Here's how the part is built. I have some questions about the finished solid (model axes, mm). Face numbers are marked on the shaded views. A direction names the side the tool comes from. Coordinates: 2 decimals unless noted, no trailing zeros. Order: outer loops, then holes, each group sorted by start corner. A loop starts at its lowest first (then second) coordinate and runs counter-clockwise, first axis right, second up. Notation, with made-up numbers: (18, 57.5) - (31, 57.5) arc R29 ccw to (31, 85.5) - close; hole circle Ø10 at (60.25, 15). An arc over 180 degrees is marked (long way). Answer as CSV lines item,"result". Start each with the question number.
Item 1: I need wall thicknesses on line 1 (X direction, y = 1.2, z = 4.5) (3 decimals); line 2 (X direction, y = 1.45, z = 31.5) (3 decimals); line 3 (X direction, y = 10.5, z = 6.5). Which ranges of each line are inside material? Lowest first, please.
Item 2: On a 3-axis mill with a long thin cutter (end or side, diameter ignored), from which of +Z, -Z, +X, -X, +Y, -Y can I reach the whole of each face in a straight line? I mean the marked faces 1, 2, 3 and 4. Say none if no direction works.
Item 3: Imagine slicing it at C-C on x = 4.5. List the corners of the cut face in (y, z) for me (3 decimals).
Item 4: Imagine slicing it at A-A on z = 29. List the corners of the cut face in (x, y) for me, and give its area (3 significant figures).
Item 5: I'm going to push flat-ended pins straight in: pin 1 (3.5 mm diameter, centred on y = 7.5, z = 18, fed in from +X); pin 2 (1.5 mm diameter, centred on y = 7, z = 6.5, fed in from -X); pin 3 (3.5 mm diameter, centred on x = 36, z = 11, fed in from +Y); pin 4 (1.5 mm diameter, centred on x = 29.5, y = 2, fed in from -Z). Where does each tip first touch, or does it pass through?
Item 6: Imagine slicing it at D-D on z = 16. List the corners of the cut face in (x, y) for me.
Item 7: We'd pull the mould along X, two halves only. Please class the marked faces 5 and 6: pulls with the +X half, pulls with the -X half, needs draft (parallel to the pull), parting line crosses it, or undercut.
Item 8: Imagine slicing it at B-B on y = 7.5. List the corners of the cut face in (x, z) for me.
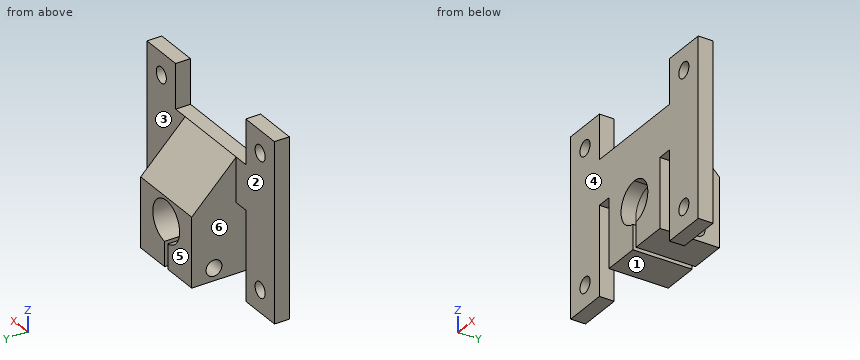
from build123d import *

# Parameters (mm, degrees)
SKETCH2_R           = 1.575
BOSS_EXTRUDE4_DEPTH = 3
BOSS_EXTRUDE5_DEPTH = 9
RIB2_REACH          = 44.895
SKETCH8_WALL_W      = 100.51836442
SKETCH8_WALL_H      = 16
SKETCH9_R           = 1.6
CUT_EXTRUDE1_DEPTH  = 48.15930449


with BuildPart() as part:
    # Sketch2 → Boss-Extrude4 (new body)
    # profile 1 of 4: a face of its own
    with BuildSketch(Plane(origin=(0, 0, 0), x_dir=(1, 0, 0), z_dir=(0, 1, 0))):
        Polygon((28, -18), (20, -18), (20, -27), (31, -27), (31, -36), (40, -36), (40, 0), (31, 0), (31, -18), align=None)
        with Locations(Location((35.5, -31.5, 0), (0, 0, 270))):
            Circle(SKETCH2_R, mode=Mode.SUBTRACT)
        with Locations(Location((35.5, -4.5, 0), (0, 0, 270))):
            Circle(SKETCH2_R, mode=Mode.SUBTRACT)
    # profile 2 of 4: a face of its own
    with BuildSketch(Plane(origin=(0, 0, 0), x_dir=(1, 0, 0), z_dir=(0, 1, 0))):
        Polygon((9, 0), (0, 0), (0, -36), (9, -36), (9, -27), (20, -27), (20, -18), (12, -18), (9, -18), align=None)
        with Locations(Location((4.5, -31.5, 0), (0, 0, 270))):
            Circle(SKETCH2_R, mode=Mode.SUBTRACT)
        with Locations(Location((4.5, -4.5, 0), (0, 0, 270))):
            Circle(SKETCH2_R, mode=Mode.SUBTRACT)
    # profile 3 of 4: a face of its own
    with BuildSketch(Plane(origin=(0, 0, 0), x_dir=(1, 0, 0), z_dir=(0, 1, 0))):
        with BuildLine():
            Line((20, -17.370131892), (20, -18))
            Line((20, -18), (28, -18))
            Line((28, -18), (28, -4))
            Line((28, -4), (20.5, -4))
            Line((20.5, -4), (20.5, -9))
            ThreePointArc((20.5, -9), (24.192526324, -13.420577547), (20, -17.370131892))
        make_face()
    # profile 4 of 4: a face of its own
    with BuildSketch(Plane(origin=(0, 0, 0), x_dir=(1, 0, 0), z_dir=(0, 1, 0))):
        with BuildLine():
            Line((12, -4), (12, -18))
            Line((12, -18), (20, -18))
            Line((20, -18), (20, -17.370131892))
            ThreePointArc((20, -17.370131892), (15.807473676, -13.420577547), (19.5, -9))
            Line((19.5, -9), (19.5, -4))
            Line((19.5, -4), (12, -4))
        make_face()
    extrude(amount=BOSS_EXTRUDE4_DEPTH)

    # Sketch6 → Boss-Extrude5 (add)
    with BuildSketch(Plane(origin=(0, 3, 0), x_dir=(1, 0, 0), z_dir=(0, 1, 0))):
        with BuildLine():
            Line((12, -18), (28, -18))
            Line((28, -18), (28, -4))
            Line((28, -4), (20.5, -4))
            Line((20.5, -4), (20.5, -9))
            ThreePointArc((20.5, -9), (20, -17.370131892), (19.5, -9))
            Line((19.5, -9), (19.5, -4))
            Line((19.5, -4), (12, -4))
            Line((12, -4), (12, -18))
        make_face()
    extrude(amount=BOSS_EXTRUDE5_DEPTH)

    # Sketch8 wall → Rib2 (add, up to next)
    with BuildSketch(Plane(origin=(20, 7.5, 22.5), x_dir=(0, -0.707106781187, 0.707106781187), z_dir=(0, 0.707106781187, 0.707106781187)), mode=Mode.PRIVATE) as rib2_sk1:
        Rectangle(SKETCH8_WALL_W, SKETCH8_WALL_H)
    rib2_tool1 = extrude(rib2_sk1.sketch, amount=-RIB2_REACH, mode=Mode.PRIVATE) - part.part
    add(rib2_tool1.solids().sort_by_distance((20, 7.5, 22.5))[0])

    # Sketch9 → Cut-Extrude1 (cut, through all)
    with BuildSketch(Plane.ZY.offset(-12)):
        with Locations((6.5, 7.5)):
            Circle(SKETCH9_R)
    extrude(amount=-CUT_EXTRUDE1_DEPTH, mode=Mode.SUBTRACT)


solid = part.part
Responses:
1,line 1,"x = 0 to 2.925, 6.075 to 9, 12 to 19.5, 20.5 to 28, 31 to 33.925, 37.075 to 40"
1,line 2,"x = 0 to 2.925, 6.075 to 9, 31 to 33.925, 37.075 to 40"
1,line 3,"x = 12 to 19.5, 20.5 to 28"
2,face 1,"-Z, +Y, -Y"
2,face 2,"+Z, -Z, -X, +Y"
2,face 3,"+Z, -Z, +X, +Y"
2,face 4,"+Z, -Z, +X, -X, -Y"
3,outline,"(0, 0) - (3, 0) - (3, 2.925) - (0, 2.925) - close; (0, 6.075) - (3, 6.075) - (3, 29.925) - (0, 29.925) - close; (0, 33.075) - (3, 33.075) - (3, 36) - (0, 36) - close"
4,outline,"(0, 0) - (9, 0) - (9, 3) - (0, 3) - close; (31, 0) - (40, 0) - (40, 3) - (31, 3) - close"
4,area,"54.0 mm^2"
5,pin 1,"stops at x = 28"
5,pin 2,"passes through"
5,pin 3,"stops at y = 3"
5,pin 4,"stops at z = 18"
6,outline,"(0, 0) - (9, 0) - (9, 3) - (0, 3) - close; (12, 0) - (16.9, 0) - (16.9, 12) - (12, 12) - close; (23.1, 0) - (28, 0) - (28, 12) - (23.1, 12) - close; (31, 0) - (40, 0) - (40, 3) - (31, 3) - close"
7,face 5,"needs draft"
7,face 6,"undercut"
8,outline,"(12, 4) - (19.5, 4) - (19.5, 4.9) - (12, 4.9) - close; (12, 8.1) - (19.5, 8.1) - (19.5, 9) arc R4.2 cw (long way) to (20.5, 9) - (20.5, 8.1) - (28, 8.1) - (28, 22.5) - (12, 22.5) - close; (20.5, 4) - (28, 4) - (28, 4.9) - (20.5, 4.9) - close"
